Here's the drawing with two shaded views (mm, measured from the low corner). I have some questions. A direction names the side the tool comes from. Coordinates: 2 decimals unless noted, no trailing zeros. Write each loop counter-clockwise with the first axis right and the second up, starting at its lowest first coordinate (ties: lowest second). Pieces come first, ordered by that corner, then holes. Notation, with made-up numbers: (29.5, 74.5) - (60.5, 74.5) arc R16 ccw to (60.5, 81.5) - close; hole circle Ø5 at (54, 1). An arc over 180 degrees is marked (long way). Answer in a Markdown table with one row per item. Add a question column.
Item 1: We'd pull the mould along Z, two halves only. Please class the marked faces 1, 2, 3 and 4: +Z half, -Z half, draft (parallel to the pull), parting line (faces both ways), or undercut.
Item 2: I'm going to push flat-ended pins straight in: pin 1 (1.5 mm diameter, centred on y = 10, z = 7, fed in from +X); pin 2 (3 mm diameter, centred on x = 3.5, z = 5.5, fed in from +Y). Where does each tip first touch, or does it pass through?
Item 3: If I drill on probe 1 along Z at (x, y) = (5, 2); probe 2 along X at (y, z) = (5.25, 1.25); probe 3 along Y at (x, z) = (31, 0.5), over which ranges is the centre line in solid material (lowest first)? Write a range as from..to.
Item 4: Which directions (+Z, -Z, +X, -X, +Y, -Y) give clear straight access to the entire face, cutting with the end or side of a thin tool? Please do the marked faces 5, 6 and 7.
Item 5: Imagine slicing it at C-C (z = 1.75). Please give me the cut outline in (x, y), plus the area to 3 significant figures.
Item 6: Imagine slicing it at D-D (x = 20). Please give me the cut outline in (y, z), plus the area to 3 significant figures.
Item 7: Imagine slicing it at A-A (x = 35). Please give me the cut outline in (y, z).
Item 8: Imagine slicing it at B-B (y = 4.5). Please give me the cut outline in (x, z).
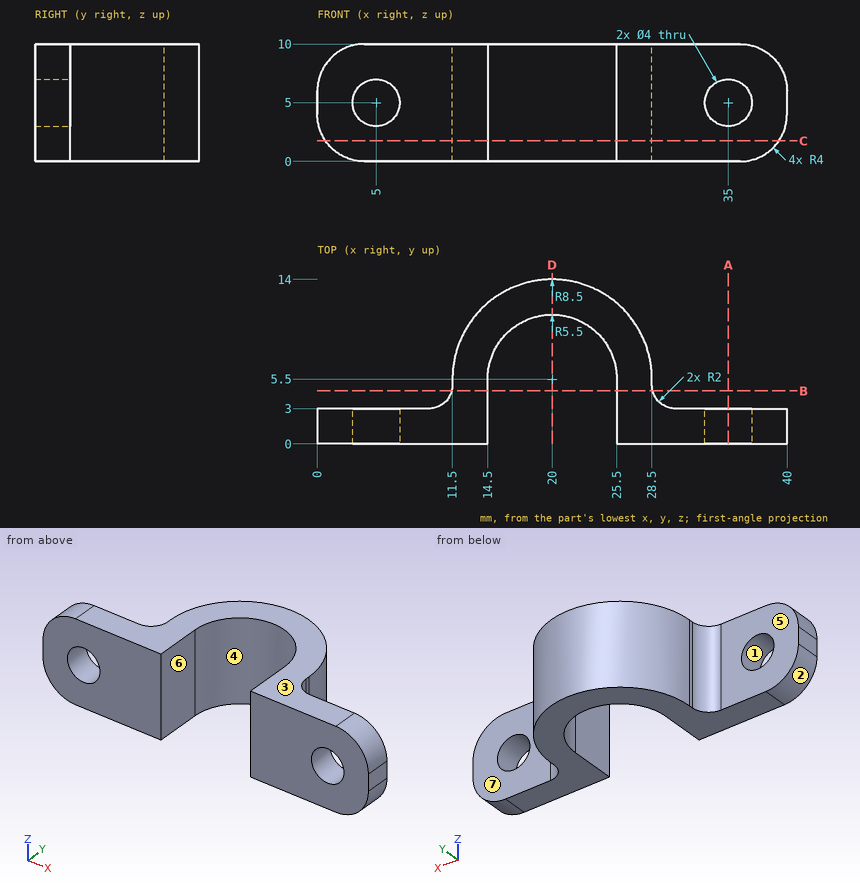
Here are the results:
| question | item | result |
|---|---|---|
| 1 | face 1 | undercut |
| 1 | face 2 | -Z half |
| 1 | face 3 | +Z half |
| 1 | face 4 | draft |
| 2 | pin 1 | stops at x = 27.63 |
| 2 | pin 2 | stops at y = 3 |
| 3 | probe 1 | z = 0..3, 7..10 |
| 3 | probe 2 | x = 11.5..14.5, 25.5..28.5 |
| 3 | probe 3 | y = 0..3 |
| 4 | face 5 | +Z, -Z, -X, +Y |
| 4 | face 6 | +Z, -Z, -Y |
| 4 | face 7 | +Z, -Z, +X, +Y |
| 5 | outline | (0.69, 0) - (14.5, 0) - (14.5, 5.5) arc R5.5 cw to (25.5, 5.5) - (25.5, 0) - (39.31, 0) - (39.31, 3) - (30.5, 3) arc R2 cw to (28.5, 5) - (28.5, 5.5) arc R8.5 ccw to (11.5, 5.5) - (11.5, 5) arc R2 cw to (9.5, 3) - (0.69, 3) - close |
| 5 | area | 166 mm2 |
| 6 | outline | (11, 0) - (14, 0) - (14, 10) - (11, 10) - close |
| 6 | area | 30.0 mm2 |
| 7 | outline | (0, 0) - (3, 0) - (3, 3) - (0, 3) - close; (0, 7) - (3, 7) - (3, 10) - (0, 10) - close |
| 8 | outline | (11.44, 0) - (14.5, 0) - (14.5, 10) - (11.44, 10) - close; (25.5, 0) - (28.56, 0) - (28.56, 10) - (25.5, 10) - close |
